from build123d import *

# Parameters (mm, degrees)
FILLET1_R            = 0.2
FILLET1_OF_MIRROR1_R = 0.2


with BuildPart() as part:
    # Sketch1 → Revolve1 (revolve)
    with BuildSketch(Plane(origin=(0, 0, 0), x_dir=(0, 0, -1), z_dir=(1, 0, 0))):
        Polygon((-4, 1.5), (-3.5, 1.5), (-3.5, 1.4), (-2.25, 1.4), (-2.25, 1.5), (-1.5, 1.5), (-1.5, 0), (-4, 0), align=None)
    revolve1 = revolve(axis=Axis((0, 17.307692308, 0), (0, -1, 0)))

    # Fillet1
    fillet1_edges = [part.edges().sort_by_distance(p)[0] for p in [
        (0, 1.5, -4),
        (0, 1.5, -1.5),
    ]]
    fillet(fillet1_edges, radius=FILLET1_R)

    # Mirror1: Revolve1 across plane
    add(revolve1.mirror(Plane.ZX))

    # Fillet1 of Mirror1
    fillet1_of_mirror1_edges = [part.edges().sort_by_distance(p)[0] for p in [
        (0, -1.5, -4),
        (0, -1.5, -1.5),
    ]]
    fillet(fillet1_of_mirror1_edges, radius=FILLET1_OF_MIRROR1_R)


solid = part.part
Work out the finished part from the listing and answer in its coordinate system (mm). Give positions to 0.01 mm unless a question says otherwise; leave off trailing zeros. Loops run counter-clockwise (first coordinate to the right, second up) from the corner with the lowest first, then second, coordinate; pieces in that order, holes last. Notation, with made-up numbers: M 62.5,-2 L 86.5,-2 A20 cw 86.5,29 Z; hole C 87,1.5 d11. An arc over 180 degrees is marked long. Use CSV: the item, a comma, the result in double quotes.
1) Consider L1, parallel to X at y = -0.55, z = 0; L2, parallel to Z at x = 1, y = 1.05. Determine where each line is inside the solid, lowest interval first.
Answer:
L1,"-4 to -1.5, 1.5 to 4"
L2,"-3.87 to -1.12, 1.12 to 3.87"
2) Find section C-C on y = 0.9. Write down the section's boundary in (x, z), plus the area to 3 significant figures.
Answer:
outline,"C 0,0 d8; hole C 0,0 d3"
area,"43.2 mm^2"
3) Determine the mould class of faces 1 (the flat face through (-2, 1.5, 0)), 2 (the flat face through (0.7, -1.4, 2.3)), 3 (the flat face through (0.7, 1.4, 2.3)) for opening direction Z: released by +Z, released by -Z, zero draft, split by the parting line, or undercut.
Answer:
face 1,"zero draft"
face 2,"undercut"
face 3,"undercut"
4) Given P1, Ø3.5, axis at x = 0.5, z = 0, coming from the -Y side, flat-ended and moving along its own axis, determine where the tip first touches the part or whether it passes through.
Answer:
P1,"y = -1.5"
